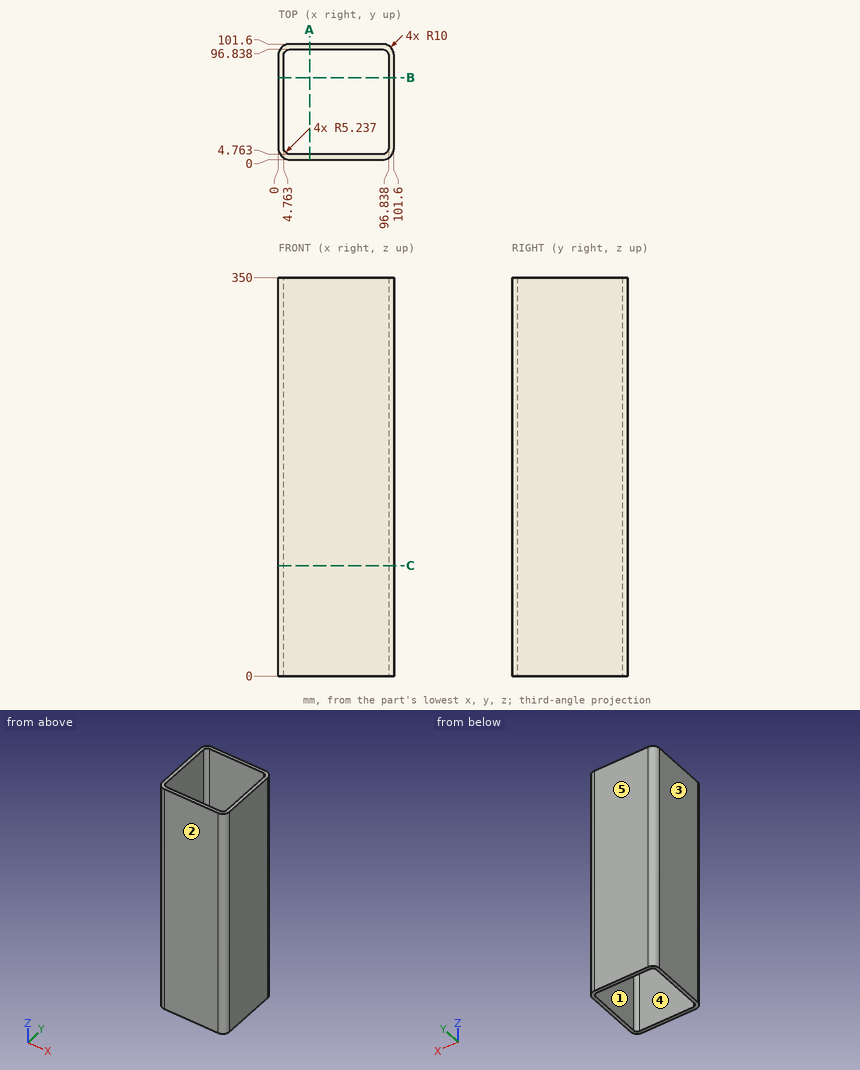
Input: dimensioned drawing with shaded views. Units: mm. Origin: part minimum x, y, z. A direction names the side the tool comes from. Coordinates: 2 decimals unless noted, no trailing zeros. Order: outer loops, then holes, each group sorted by start corner. A loop starts at its lowest first (then second) coordinate and runs counter-clockwise, first axis right, second up. Notation, with made-up numbers: (15, 19.5) - (44, 19.5) arc R16 cw to (44, 36.5) - close; hole circle Ø3 at (-10.75, 51.25). An arc over 180 degrees is marked (long way). Put each result on its own line as item: value.
1. Reachability of the marked faces 1 and 2 from +Z, -Z, +X, -X, +Y, -Y: full face, straight path, thin tool, end or side. Return the list, or none.
Report:
face 1: +Z, -Z
face 2: +Z, -Z, +X, -X, -Y
2. Cut plane C-C on z = 97. Return the cut outline in (x, y) (1 decimal).
Report:
outline: (0, 10) arc R10 ccw to (10, 0) - (91.6, 0) arc R10 ccw to (101.6, 10) - (101.6, 91.6) arc R10 ccw to (91.6, 101.6) - (10, 101.6) arc R10 ccw to (0, 91.6) - close; hole (4.8, 10) arc R5.2 ccw to (10, 4.8) - (91.6, 4.8) arc R5.2 ccw to (96.8, 10) - (96.8, 91.6) arc R5.2 ccw to (91.6, 96.8) - (10, 96.8) arc R5.2 ccw to (4.8, 91.6) - close
3. Line query: line 1 along X through (y, z) = (72.5, 254.5); line 2 along X through (y, z) = (93, 183.5). Output: solid intervals per line, ascending.
Report:
line 1: x = 0 to 4.76, 96.84 to 101.6
line 2: x = 0.1 to 4.95, 96.65 to 101.5
4. Cut plane A-A on x = 27.5. Return the cut outline in (y, z).
Report:
outline: (0, 0) - (4.76, 0) - (4.76, 350) - (0, 350) - close; (96.84, 0) - (101.6, 0) - (101.6, 350) - (96.84, 350) - close
5. Draft query along Y for the marked faces 3, 4 and 5. Return one class per face: pulls with the +Y half, pulls with the -Y half, needs draft (parallel to the pull), parting line crosses it, or undercut.
Report:
face 3: needs draft
face 4: undercut
face 5: pulls with the +Y half
